```python
from build123d import *

# Parameters (mm, degrees)
EXTRUDE_1_DEPTH     = 2
SKETCH_3_R          = 2.75
SKETCH_3_R_2        = 1.75
SKETCH_3_R_3        = 11.5
CUT_EXTRUDE_1_DEPTH = 3


with BuildPart() as part:
    # 草图1 → 凸台-拉伸1 (new body)
    with BuildSketch(Plane(origin=(0, 0, 0), x_dir=(1, 0, 0), z_dir=(0, 1, 0))):
        Polygon((-63, 0), (-63, -63), (0, -63), (0, -21), (-21, -21), (-21, 0), align=None)
    extrude(amount=EXTRUDE_1_DEPTH)

    # 草图3 → 切除-拉伸1 (cut, through all)
    with BuildSketch(Plane(origin=(0, 2, 0), x_dir=(1, 0, 0), z_dir=(0, 1, 0))):
        with Locations((-53, -10)):
            Circle(SKETCH_3_R)
        with Locations((-56.5, -56.5)):
            Circle(SKETCH_3_R_2)
        with Locations((-25.5, -56.5)):
            Circle(SKETCH_3_R_2)
        with Locations((-25.5, -25.5)):
            Circle(SKETCH_3_R_2)
        with Locations((-56.5, -25.5)):
            Circle(SKETCH_3_R_2)
        with Locations((-41, -41)):
            Circle(SKETCH_3_R_3)
        with Locations((-10, -53)):
            Circle(SKETCH_3_R)
        with Locations((-10, -31)):
            Circle(SKETCH_3_R)
        with Locations((-31, -10)):
            Circle(SKETCH_3_R)
        Polygon((-63, -63), (-63, -55.928932188), (-55.928932188, -63), align=None)
    extrude(amount=-CUT_EXTRUDE_1_DEPTH, mode=Mode.SUBTRACT)


solid = part.part
```
Source: CAD feature listing. Evaluate the final solid. Frame: model axes, mm. A direction names the side the tool comes from. Round coordinates to 2 decimals unless told otherwise and drop trailing zeros. Loops run counter-clockwise (first coordinate to the right, second up) from the corner with the lowest first, then second, coordinate; pieces in that order, holes last.
(1) Section query D-D (x = -41). Output: boundary loops of the cut face in (y, z), and give its area (3 significant figures).
From the geometry:
outline: (0, 0) - (2, 0) - (2, 29.5) - (0, 29.5) - close; (0, 52.5) - (2, 52.5) - (2, 63) - (0, 63) - close
area: 80.0 mm2
(2) Section query B-B (y = 0.9). Give the number of separate pieces and of enclosed holes in the cut face, and give its area (3 significant figures).
From the geometry:
separate pieces: 1
enclosed holes: 9
area: 2,950 mm2
(3) Contact query for flat-ended pins moving along their axis: pin 1 Ø2 at (x, z) = (-25.5, 25.5) entering from -Y; pin 2 Ø5.5 at (x, z) = (-56.5, 25.5) entering from -Y; pin 3 Ø1 at (x, y) = (-6.5, 1) entering from -Z. Output: stop coordinate, or through.
From the geometry:
pin 1: passes through
pin 2: stops at y = 0
pin 3: stops at z = 21
(4) Section query C-C (z = 43.5). Output: boundary loops of the cut face in (x, y), and give its area (3 significant figures).
From the geometry:
outline: (-63, 0) - (-52.22, 0) - (-52.22, 2) - (-63, 2) - close; (-29.78, 0) - (0, 0) - (0, 2) - (-29.78, 2) - close
area: 81.1 mm2
(5) Access query for faces 1 (the flat face through (-10, 1, 21)), 2 (the flat face through (-32, 2, 31)). Directions: +Z, -Z, +X, -X, +Y, -Y. A direction counts if a zero-diameter tool reaches every point of the face in a straight line with its end or side. Return the directions, or none.
From the geometry:
face 1: -Z, +X, +Y, -Y
face 2: +Z, -Z, +X, -X, +Y
(6) Material intervals for probe 1 along X at (y, z) = (0.5, 10); probe 2 along Z at (x, y) = (-25.5, 1.25); probe 3 along X at (y, z) = (0.7, 41), sorted ascending.
From the geometry:
probe 1: x = -63 to -55.75, -50.25 to -33.75, -28.25 to -21
probe 2: z = 0 to 23.75, 27.25 to 54.75, 58.25 to 63
probe 3: x = -63 to -52.5, -29.5 to 0
(7) Pull-direction query (X, two-part tool) for faces 3 (the flat face through (-63, 1, 28)), 4 (the flat face through (-28, 1, 63)), 5 (the flat face through (-21, 1, 11)), 6 (the cylindrical face through (-54.883, 1.014, 57.17)); classes: +X half, -X half, draft (parallel to the pull), parting line (faces both ways), or undercut.
From the geometry:
face 3: -X half
face 4: draft
face 5: +X half
face 6: undercut
(8) Section query A-A (x = -25.5). Output: boundary loops of the cut face in (y, z).
From the geometry:
outline: (0, 0) - (2, 0) - (2, 23.75) - (0, 23.75) - close; (0, 27.25) - (2, 27.25) - (2, 54.75) - (0, 54.75) - close; (0, 58.25) - (2, 58.25) - (2, 63) - (0, 63) - close
